```python
from build123d import *

# Parameters (mm, degrees)
RESSALTO_EXTRUS_O1_DEPTH      = 4.2
RESSALTO_EXTRUS_O1_DEPTH_BACK = 30
ESBO_O1_R                     = 6.0125
ESBO_O1_R_2                   = 4.7625
ESBO_O2_R                     = 9.0125
ESBO_O2_R_2                   = 6.0125
RESSALTO_EXTRUS_O2_DEPTH      = 4.2
FILETE2_R                     = 0.5


with BuildPart() as part:
    # Esboço1 → Ressalto-extrusão1 (new, two sides: drawn at the far end of the back side and taken through both)
    with BuildSketch(Plane.XY.offset(-0.404551317).offset(-RESSALTO_EXTRUS_O1_DEPTH_BACK)):
        with Locations((70.795334041, 51.25825559)):
            Circle(ESBO_O1_R)
        with Locations((70.795334041, 51.25825559)):
            Circle(ESBO_O1_R_2, mode=Mode.SUBTRACT)
    extrude(amount=RESSALTO_EXTRUS_O1_DEPTH + RESSALTO_EXTRUS_O1_DEPTH_BACK)

    # Esboço2 → Ressalto-extrusão2 (add)
    with BuildSketch(Plane.XY.offset(-0.404551317)):
        with Locations((70.795334041, 51.25825559)):
            Circle(ESBO_O2_R)
        with Locations((70.795334041, 51.25825559)):
            Circle(ESBO_O2_R_2, mode=Mode.SUBTRACT)
    extrude(amount=RESSALTO_EXTRUS_O2_DEPTH)

    # Filete2
    filete2_edges = [part.edges().sort_by_distance(p)[0] for p in [
        (61.782834041, 51.25825559, 3.795448683),
        (61.782834041, 51.25825559, -0.404551317),
        (64.782834041, 51.25825559, -30.404551317),
    ]]
    fillet(filete2_edges, radius=FILETE2_R)


solid = part.part
```
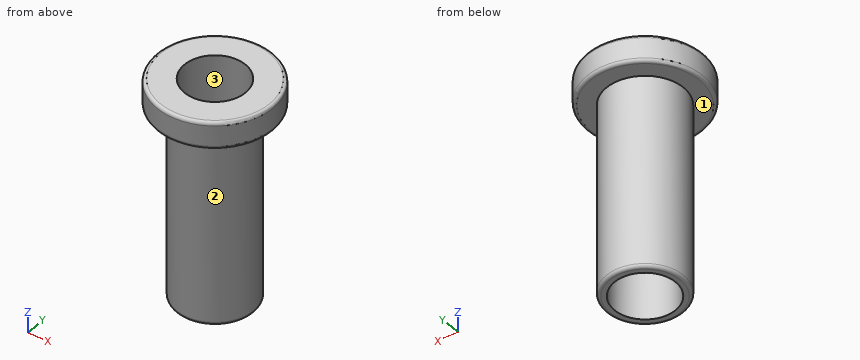
Geometry: final body of the model. Coordinates: model frame, mm. Face numbers are marked on the shaded views. Give positions to 0.01 mm unless a question says otherwise; leave off trailing zeros. Loops run counter-clockwise (first coordinate to the right, second up) from the corner with the lowest first, then second, coordinate; pieces in that order, holes last. Notation, with made-up numbers: (65, 51) -> (81, 51) arc R22 ccw to (81, 82) -> close; hole circle Ø9 at (55, -21.75). An arc over 180 degrees is marked (long way). Return JSON: item names as keys, results as strings.
Item 1: Pin query (flat end, axial travel): P1, Ø1, axis at x = 65, z = -25.5, coming from the +Y side; P2, Ø2, axis at y = 47.5, z = -17.5, coming from the -X side; P3, Ø4, axis at y = 58.5, z = -15, coming from the +X side. Return the tip coordinate at first contact, or that it passes through.
Filled in:
{"P1": "y = 54.11", "P2": "x = 65.45", "P3": "x = 73.74"}
Item 2: Mould query, pull axis X, two halves, no side actions, for the marked faces 1, 2 and 3. Classes: released by +X, released by -X, zero draft, split by the parting line, or undercut.
Filled in:
{"face 1": "zero draft", "face 2": "split by the parting line", "face 3": "undercut"}
Item 3: Section A-A, the plane z = -1.5. Output: boundary loops of the cut face in (x, y) (1 decimal), plus the area to 3 significant figures.
Filled in:
{"outline": "circle Ø12 at (70.8, 51.3); hole circle Ø9.5 at (70.8, 51.3)", "area": "42.3 mm^2"}
Item 4: Line query: line 1 (Y direction, x = 71, z = -0.5); line 2 (X direction, y = 47.25, z = -1); line 3 (Z direction, x = 67, y = 56). Output: solid intervals per line, ascending.
Filled in:
{"line 1": "45.25 to 46.5, 56.02 to 57.27", "line 2": "66.31 to 68.22, 73.37 to 75.28", "line 3": "-0.4 to 3.8"}
